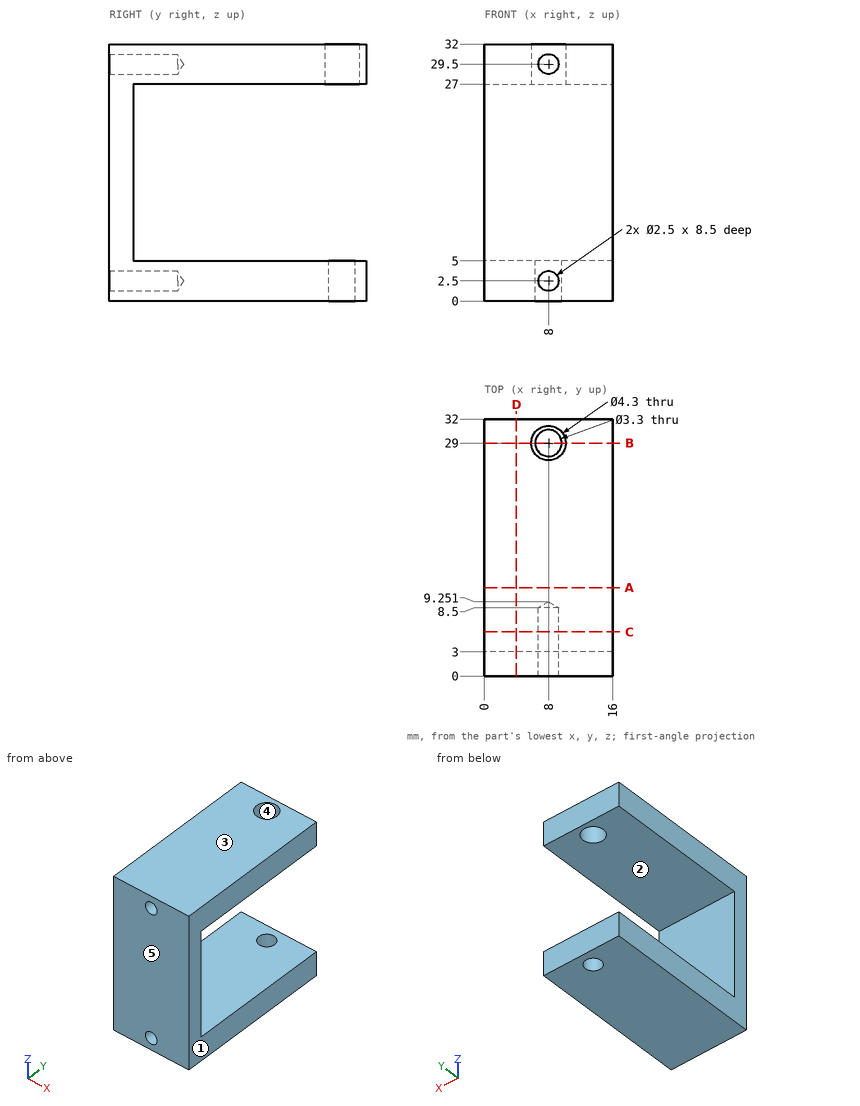
Drawing for the job (mm, zero at the part's lowest x, y, z). A direction names the side the tool comes from. Give positions to 0.01 mm unless a question says otherwise; leave off trailing zeros. Loops run counter-clockwise (first coordinate to the right, second up) from the corner with the lowest first, then second, coordinate; pieces in that order, holes last. Notation, with made-up numbers: M -27.5,88.25 L -6.5,88.25 A33 cw -6.5,123.25 Z; hole C 39,48 d8. An arc over 180 degrees is marked long. Use one line per item in the form item = value.
Item 1: Flat gauge pins, fed straight in: pin 1 (2 mm diameter, centred on x = 3, z = 9.5, fed in from +Y); pin 2 (2 mm diameter, centred on x = 8, z = 29.5, fed in from -Y). Where does each tip first touch, or does it go through?
Determined:
pin_1 = 3
pin_2 = 8.65
Item 2: Slice it at D-D (x = 4). List the corners of the cut face in (y, z).
Determined:
outline = M 0,0 L 32,0 L 32,5 L 3,5 L 3,27 L 32,27 L 32,32 L 0,32 Z
Item 3: Slice it at B-B (y = 29). List the corners of the cut face in (x, z), plus the area to 3 significant figures.
Determined:
outline = M 0,0 L 6.35,0 L 6.35,5 L 0,5 Z; M 0,27 L 5.85,27 L 5.85,32 L 0,32 Z; M 9.65,0 L 16,0 L 16,5 L 9.65,5 Z; M 10.15,27 L 16,27 L 16,32 L 10.15,32 Z
area = 122 mm2
Item 4: Slice it at C-C (y = 5.5). List the corners of the cut face in (x, z), plus the area to 3 significant figures.
Determined:
outline = M 0,0 L 16,0 L 16,5 L 0,5 Z; M 0,27 L 16,27 L 16,32 L 0,32 Z; hole C 8,2.5 d2.5; hole C 8,29.5 d2.5
area = 150 mm2
Item 5: Drill centre lines: probe 1 along Z at (x, y) = (8, 6.25); probe 2 along Z at (x, y) = (7, 12); probe 3 along X at (y, z) = (3, 2.5). Where is each one in solid material? Low to high. Write a range as from..to.
Determined:
probe_1 = 0..1.25, 3.75..5, 27..28.25, 30.75..32
probe_2 = 0..5, 27..32
probe_3 = 0..6.75, 9.25..16
Item 6: Slice it at A-A (y = 11). List the corners of the cut face in (x, z).
Determined:
outline = M 0,0 L 16,0 L 16,5 L 0,5 Z; M 0,27 L 16,27 L 16,32 L 0,32 Z
Item 7: Two-plate mould, pull along Y, no slides. Class the marked faces 3, 4 and 5: pulls with the +Y half, pulls with the -Y half, needs draft (parallel to the pull), parting line crosses it, or undercut.
Determined:
face_3 = needs draft
face_4 = undercut
face_5 = pulls with the -Y half
Item 8: Which spindle directions (+Z, -Z, +X, -X, +Y, -Y) get a long thin tool onto all of the face, cutting with end or side? Do the marked faces 1 and 2. Say none if no direction does.
Determined:
face_1 = +Z, -Z, +X, +Y, -Y
face_2 = +X, -X, +Y
